```python
from build123d import *

# Parameters (mm, degrees)
SKETCH_1_R          = 5
EXTRUDE_1_DEPTH     = 15.5
SKETCH_2_R          = 6
EXTRUDE_2_DEPTH     = 17.91
CUT_EXTRUDE_1_DEPTH = 2
SKETCH_4_R          = 5
EXTRUDE_3_DEPTH     = 7
SKETCH_5_R          = 7
EXTRUDE_4_DEPTH     = 1
SKETCH_6_R          = 6
EXTRUDE_5_DEPTH     = 6
CUT_EXTRUDE_2_DEPTH = 2
SKETCH_8_R          = 1.25
CUT_EXTRUDE_3_DEPTH = 10
EXTRUDE_START       = 1
SKETCH_9_R          = 7
EXTRUDE_6_DEPTH     = 1
CUT_EXTRUDE_START   = -1
SKETCH_10_R         = 7
SKETCH_10_R_2       = 6
CUT_EXTRUDE_5_DEPTH = 1


with BuildPart() as part:
    # 草图1 → 凸台-拉伸1 (new body)
    with BuildSketch(Plane.XY):
        Circle(SKETCH_1_R)
    extrude(amount=EXTRUDE_1_DEPTH)

    # 草图2 → 凸台-拉伸2 (add)
    with BuildSketch(Plane(origin=(0, 0, 0), x_dir=(-1, 0, 0), z_dir=(0, 0, -1))):
        Circle(SKETCH_2_R)
    extrude(amount=EXTRUDE_2_DEPTH)

    # 草图3 → 切除-拉伸1 (cut)
    with BuildSketch(Plane(origin=(5, 0, 0), x_dir=(0, 0, -1), z_dir=(1, 0, 0))):
        with BuildLine():
            Line((-10.75, 1.5), (-4.75, 1.5))
            ThreePointArc((-4.75, 1.5), (-3.25, 0), (-4.75, -1.5))
            Line((-4.75, -1.5), (-10.75, -1.5))
            ThreePointArc((-10.75, -1.5), (-12.25, 0), (-10.75, 1.5))
        make_face()
    extrude(amount=-CUT_EXTRUDE_1_DEPTH, mode=Mode.SUBTRACT)

    # 草图4 → 凸台-拉伸3 (add)
    with BuildSketch(Plane.XY.offset(15.5)):
        Circle(SKETCH_4_R)
    extrude(amount=EXTRUDE_3_DEPTH)

    # 草图5 → 凸台-拉伸4 (add)
    with BuildSketch(Plane(origin=(0, 0, -17.91), x_dir=(-1, 0, 0), z_dir=(0, 0, -1))):
        Circle(SKETCH_5_R)
    extrude(amount=EXTRUDE_4_DEPTH)

    # 草图6 → 凸台-拉伸5 (add)
    with BuildSketch(Plane(origin=(0, 0, -18.91), x_dir=(-1, 0, 0), z_dir=(0, 0, -1))):
        Circle(SKETCH_6_R)
    extrude(amount=EXTRUDE_5_DEPTH)

    # 草图7 → 切除-拉伸2 (cut)
    with BuildSketch(Plane(origin=(6, 0, 0), x_dir=(0, 0, -1), z_dir=(1, 0, 0))):
        with BuildLine():
            Line((20.91, 1.5), (24.91, 1.5))
            ThreePointArc((24.91, 1.5), (26.41, 0), (24.91, -1.5))
            Line((24.91, -1.5), (20.91, -1.5))
            ThreePointArc((20.91, -1.5), (19.41, 0), (20.91, 1.5))
        make_face()
    extrude(amount=-CUT_EXTRUDE_2_DEPTH, mode=Mode.SUBTRACT)

    # 草图8 → 切除-拉伸3 (cut)
    with BuildSketch(Plane(origin=(0, 0, -24.91), x_dir=(-1, 0, 0), z_dir=(0, 0, -1))):
        Circle(SKETCH_8_R)
    extrude(amount=-CUT_EXTRUDE_3_DEPTH, mode=Mode.SUBTRACT)

    # 草图9 → 凸台-拉伸6 (add)
    with BuildSketch(Plane.XY.offset(-10.47).offset(EXTRUDE_START)):
        with Locations(Location((0, 0, 0), (0, 0, 180))):
            Circle(SKETCH_9_R)
    extrude(amount=-EXTRUDE_6_DEPTH)

    # 草图10 → 切除-拉伸5 (cut)
    with BuildSketch(Plane(origin=(0, 0, -18.91), x_dir=(-1, 0, 0), z_dir=(0, 0, -1)).offset(CUT_EXTRUDE_START)):
        with Locations(Location((0, 0, 0), (0, 0, 180))):
            Circle(SKETCH_10_R)
        with Locations(Location((0, 0, 0), (0, 0, 180))):
            Circle(SKETCH_10_R_2, mode=Mode.SUBTRACT)
    extrude(amount=CUT_EXTRUDE_5_DEPTH, mode=Mode.SUBTRACT)


solid = part.part
```
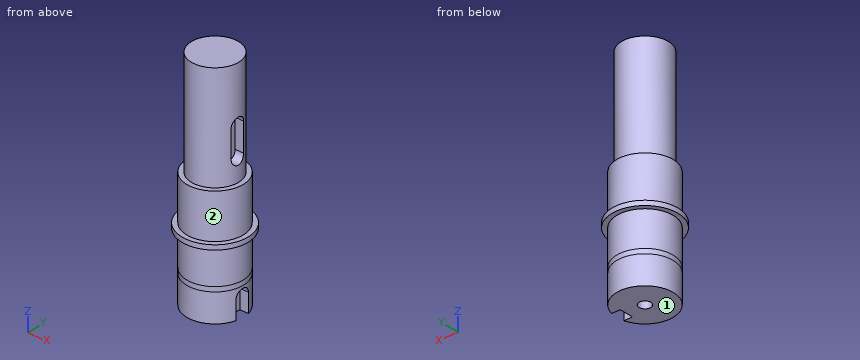
The listing builds one solid part. Answer for the finished solid, in the listing's coordinates (mm). Face numbers are marked on the shaded views. A direction names the side the tool comes from. Round coordinates to 2 decimals unless told otherwise and drop trailing zeros. Loops run counter-clockwise (first coordinate to the right, second up) from the corner with the lowest first, then second, coordinate; pieces in that order, holes last.
1) A cutting plane is placed at C-C on z = 8.5. Determine the outline of the cut face in (x, y), plus the area to 3 significant figures.
Outcome:
outline: (3, -1.5) - (3, 1.5) - (4.77, 1.5) arc R5 ccw (long way) to (4.77, -1.5) - close
area: 72.8 mm2
2) A cutting plane is placed at A-A on y = 0. Determine the outline of the cut face in (x, z).
Outcome:
outline: (-7, -10.47) - (-6, -10.47) - (-6, -24.91) - (-1.25, -24.91) - (-1.25, -14.91) - (1.25, -14.91) - (1.25, -24.91) - (4, -24.91) - (4, -19.41) - (6, -19.41) - (6, -10.47) - (7, -10.47) - (7, -9.47) - (6, -9.47) - (6, 0) - (5, 0) - (5, 3.25) - (3, 3.25) - (3, 12.25) - (5, 12.25) - (5, 22.5) - (-5, 22.5) - (-5, 0) - (-6, 0) - (-6, -9.47) - (-7, -9.47) - close
3) Given P1, Ø0.5, axis at x = 3.5, z = 9, coming from the +Y side; P2, Ø2, axis at y = 0.5, z = -15, coming from the -X side; P3, Ø3.5, axis at y = 0, z = 7, coming from the +X side; P4, Ø1.5, axis at x = -4.5, y = -3.5, coming from the +Z side, each flat-ended and moving along its own axis, determine where each tip first touches the part or whether it passes through.
Outcome:
P1: stops at y = 3.8
P2: stops at x = -6
P3: stops at x = 4.77
P4: stops at z = 22.5
4) A cutting plane is placed at D-D on y = -5.5. Determine the outline of the cut face in (x, z), plus the area to 3 significant figures.
Outcome:
outline: (-4.33, -10.47) - (-2.4, -10.47) - (-2.4, -24.91) - (2.4, -24.91) - (2.4, -10.47) - (4.33, -10.47) - (4.33, -9.47) - (2.4, -9.47) - (2.4, 0) - (-2.4, 0) - (-2.4, -9.47) - (-4.33, -9.47) - close
area: 123 mm2
5) Consider line 1 (Y direction, x = 0, z = -20.25); line 2 (Z direction, x = 3, y = -5.25); line 3 (Y direction, x = 0, z = 16.5). Determine where each line is inside the solid, lowest interval first.
Outcome:
line 1: y = -6 to -1.25, 1.25 to 6
line 2: z = -10.47 to -9.47
line 3: y = -5 to 5
6) For the marked faces 1 and 2, determine the directions among +Z, -Z, +X, -X, +Y, -Y from which every point of the face is accessible in a straight line to the end or side of a thin tool.
Outcome:
face 1: -Z, +X, -X, +Y, -Y
face 2: +Z
7) A cutting plane is placed at B-B on x = 0. Determine the outline of the cut face in (y, z).
Outcome:
outline: (-7, -10.47) - (-6, -10.47) - (-6, -24.91) - (-1.25, -24.91) - (-1.25, -14.91) - (1.25, -14.91) - (1.25, -24.91) - (6, -24.91) - (6, -10.47) - (7, -10.47) - (7, -9.47) - (6, -9.47) - (6, 0) - (5, 0) - (5, 22.5) - (-5, 22.5) - (-5, 0) - (-6, 0) - (-6, -9.47) - (-7, -9.47) - close
